Can you work these out from the model? Positions are in its coordinate system, mm. A direction names the side the tool comes from. Give positions to 0.01 mm unless a question says otherwise; leave off trailing zeros. Loops run counter-clockwise (first coordinate to the right, second up) from the corner with the lowest first, then second, coordinate; pieces in that order, holes last.
from build123d import *

# Parameters (mm, degrees)
F2_DEPTH = 9
F3_DEPTH = 9


with BuildPart() as f1:
    # F0 (on Front) → F1 (revolve)
    with BuildSketch(Plane.XZ):
        Polygon((0, -50), (0, 107), (-3, 107), (-3, 92), (-4, 92), (-4, -35), (-3, -35), (-3, -50), align=None)
    revolve(axis=Axis((0, 0, 0), (0, 0, -1)))

    # F2 (add): a face of the model
    f2_faces = [f1.faces().sort_by_distance(p)[0] for p in [
        (0, 0, 107),
    ]]
    extrude(f2_faces, amount=F2_DEPTH)

    # F3 (add): a face of the model
    f3_faces = [f1.faces().sort_by_distance(p)[0] for p in [
        (0, 0, -50),
    ]]
    extrude(f3_faces, amount=F3_DEPTH)


solid = f1.part
(1) Suppose I cut it at C-C on z = 105. List the corners of the cut face in (x, y) for me.
Returned:
outline: circle Ø6 at (0, 0)
(2) Which directions (+Z, -Z, +X, -X, +Y, -Y) give clear straight access to the entire face, cutting with the end or side of a thin tool? Please do faces 1 (the flat face through (-1, 3, -35)), 2 (the flat face through (1, 3, 92)), 3 (the flat face through (0, 0, -59)).
Returned:
face 1: -Z
face 2: +Z
face 3: -Z, +X, -X, +Y, -Y
(3) Will these pins go through, and if not, where does the flat tip stop? P1, Ø2, axis at y = -3, z = 81, coming from the -X side; P2, Ø2, axis at x = -3, z = -18.5, coming from the -Y side; P3, Ø2, axis at x = 2, z = -23.5, coming from the -Y side.
Returned:
P1: stops at x = -3.46
P2: stops at y = -3.46
P3: stops at y = -3.87
(4) Suppose I cut it at D-D on z = -22.5. List the corners of the cut face in (x, y) for me.
Returned:
outline: circle Ø8 at (0, 0)
(5) Please list where these lines run through material, in increasing order: probe 1 along Y at (x, z) = (0.25, -9); probe 2 along Z at (x, y) = (-2.75, 2.5); probe 3 along X at (y, z) = (-0.5, -20).
Returned:
probe 1: y = -3.99 to 3.99
probe 2: z = -35 to 92
probe 3: x = -3.97 to 3.97
(6) Suppose I cut it at A-A on y = 0. List the corners of the cut face in (x, z) for me, plus the area to 3 significant figures.
Returned:
outline: (-4, -35) - (-3, -35) - (-3, -59) - (3, -59) - (3, -35) - (4, -35) - (4, 92) - (3, 92) - (3, 116) - (-3, 116) - (-3, 92) - (-4, 92) - close
area: 1,300 mm2
